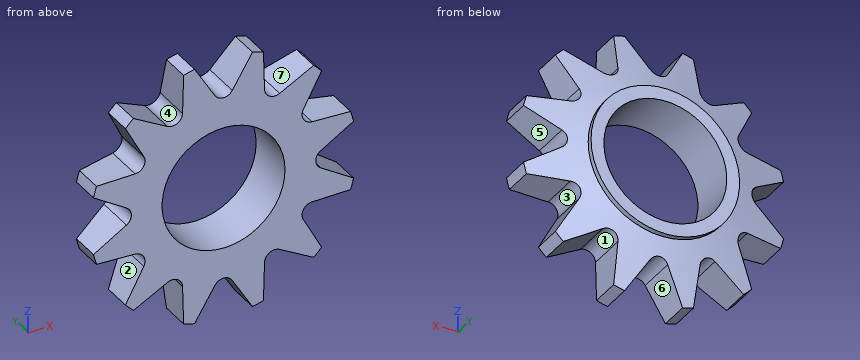
from build123d import *

# Parameters (mm, degrees)
SKETCH1_R               = 260
SKETCH1_R_2             = 120
BOSS_EXTRUDE1_DEPTH     = 45
SKETCH2_R               = 145
SKETCH2_R_2             = 120
BOSS_EXTRUDE3_DEPTH     = 55
CUT_EXTRUDE1_DEPTH      = 56
CUT_EXTRUDE1_DEPTH_BACK = 46
SCALE2_SCALE            = 0.4


with BuildPart() as part:
    # Sketch1 → Boss-Extrude1 (new body, symmetric)
    with BuildSketch(Plane(origin=(0, 0, 0), x_dir=(1, 0, 0), z_dir=(0, 1, 0))):
        Circle(SKETCH1_R)
        Circle(SKETCH1_R_2, mode=Mode.SUBTRACT)
    extrude(amount=BOSS_EXTRUDE1_DEPTH, both=True)

    # Sketch2 → Boss-Extrude3 (add)
    with BuildSketch(Plane(origin=(0, 0, 0), x_dir=(1, 0, 0), z_dir=(0, 1, 0))):
        Circle(SKETCH2_R)
        Circle(SKETCH2_R_2, mode=Mode.SUBTRACT)
    extrude(amount=BOSS_EXTRUDE3_DEPTH)

    # Sketch4 → Cut-Extrude1 (cut, two sides)
    with BuildSketch(Plane(origin=(0, 0, 0), x_dir=(1, 0, 0), z_dir=(0, 1, 0))) as cut_extrude1_sk:
        with BuildLine():
            Line((-17.033179487, 189.518072861), (-56.573051576, 253.770545642))
            ThreePointArc((-56.573051576, 253.770545642), (0, 260), (56.573051576, 253.770545642))
            Line((56.573051576, 253.770545642), (17.033179487, 189.518072861))
            ThreePointArc((17.033179487, 189.518072861), (0, 180), (-17.033179487, 189.518072861))
        make_face()
        with BuildLine():
            Line((109.510202574, 155.61087583), (175.878972656, 191.48521347))
            ThreePointArc((175.878972656, 191.48521347), (130, 225.166604984), (77.891572987, 248.058265046))
            Line((77.891572987, 248.058265046), (80.007870288, 172.644055317))
            ThreePointArc((80.007870288, 172.644055317), (90, 155.884572681), (109.510202574, 155.61087583))
        make_face()
        with BuildLine():
            Line((172.644055318, 80.007870287), (248.058265047, 77.891572986))
            ThreePointArc((248.058265047, 77.891572986), (225.166604985, 130), (191.485213471, 175.878972655))
            Line((191.485213471, 175.878972655), (155.610875831, 109.510202573))
            ThreePointArc((155.610875831, 109.510202573), (155.884572682, 90), (172.644055318, 80.007870287))
        make_face()
        with BuildLine():
            Line((189.518072862, -17.033179488), (253.770545643, -56.573051577))
            ThreePointArc((253.770545643, -56.573051577), (260.000000001, -1e-09), (253.770545643, 56.573051575))
            Line((253.770545643, 56.573051575), (189.518072862, 17.033179486))
            ThreePointArc((189.518072862, 17.033179486), (180.000000001, -1e-09), (189.518072862, -17.033179488))
        make_face()
        with BuildLine():
            Line((155.610875831, -109.510202575), (191.485213471, -175.878972657))
            ThreePointArc((191.485213471, -175.878972657), (225.166604985, -130.000000001), (248.058265047, -77.891572988))
            Line((248.058265047, -77.891572988), (172.644055318, -80.007870289))
            ThreePointArc((172.644055318, -80.007870289), (155.884572682, -90.000000001), (155.610875831, -109.510202575))
        make_face()
        with BuildLine():
            Line((80.007870288, -172.644055319), (77.891572987, -248.058265048))
            ThreePointArc((77.891572987, -248.058265048), (130, -225.166604986), (175.878972656, -191.485213472))
            Line((175.878972656, -191.485213472), (109.510202574, -155.610875832))
            ThreePointArc((109.510202574, -155.610875832), (90, -155.884572683), (80.007870288, -172.644055319))
        make_face()
        with BuildLine():
            Line((-17.033179487, -189.518072863), (-56.573051576, -253.770545644))
            ThreePointArc((-56.573051576, -253.770545644), (0, -260.000000002), (56.573051576, -253.770545644))
            Line((56.573051576, -253.770545644), (17.033179487, -189.518072863))
            ThreePointArc((17.033179487, -189.518072863), (0, -180.000000002), (-17.033179487, -189.518072863))
        make_face()
        with BuildLine():
            Line((-109.510202574, -155.610875832), (-175.878972656, -191.485213472))
            ThreePointArc((-175.878972656, -191.485213472), (-130, -225.166604986), (-77.891572987, -248.058265048))
            Line((-77.891572987, -248.058265048), (-80.007870288, -172.644055319))
            ThreePointArc((-80.007870288, -172.644055319), (-90, -155.884572683), (-109.510202574, -155.610875832))
        make_face()
        with BuildLine():
            Line((-172.644055318, -80.007870289), (-248.058265047, -77.891572988))
            ThreePointArc((-248.058265047, -77.891572988), (-225.166604985, -130.000000001), (-191.485213471, -175.878972657))
            Line((-191.485213471, -175.878972657), (-155.610875831, -109.510202575))
            ThreePointArc((-155.610875831, -109.510202575), (-155.884572682, -90.000000001), (-172.644055318, -80.007870289))
        make_face()
        with BuildLine():
            Line((-189.518072862, 17.033179486), (-253.770545643, 56.573051575))
            ThreePointArc((-253.770545643, 56.573051575), (-260.000000001, -1e-09), (-253.770545643, -56.573051577))
            Line((-253.770545643, -56.573051577), (-189.518072862, -17.033179488))
            ThreePointArc((-189.518072862, -17.033179488), (-180.000000001, -1e-09), (-189.518072862, 17.033179486))
        make_face()
        with BuildLine():
            Line((-155.610875831, 109.510202573), (-191.485213471, 175.878972655))
            ThreePointArc((-191.485213471, 175.878972655), (-225.166604985, 130), (-248.058265047, 77.891572986))
            Line((-248.058265047, 77.891572986), (-172.644055318, 80.007870287))
            ThreePointArc((-172.644055318, 80.007870287), (-155.884572682, 90), (-155.610875831, 109.510202573))
        make_face()
        with BuildLine():
            Line((-80.007870288, 172.644055317), (-77.891572987, 248.058265046))
            ThreePointArc((-77.891572987, 248.058265046), (-130, 225.166604984), (-175.878972656, 191.48521347))
            Line((-175.878972656, 191.48521347), (-109.510202574, 155.61087583))
            ThreePointArc((-109.510202574, 155.61087583), (-90, 155.884572681), (-80.007870288, 172.644055317))
        make_face()
    extrude(amount=CUT_EXTRUDE1_DEPTH, mode=Mode.SUBTRACT)
    extrude(cut_extrude1_sk.sketch, amount=-CUT_EXTRUDE1_DEPTH_BACK, mode=Mode.SUBTRACT)

    # Sketch9 → Cut-Revolve2 (revolve, cut)
    with BuildSketch(Plane(origin=(0, 0, 0), x_dir=(0, 0, -1), z_dir=(1, 0, 0))):
        Polygon((145, 45), (312.942286341, 45), (312.942286341, 0), align=None)
    revolve(axis=Axis((0, 0, 0), (0, 1, 0)), mode=Mode.SUBTRACT)


with BuildPart() as part_1:
    # Scale2: scaled about (-4.97e-06, -3.05192852, -9e-09)
    add(part.part.scale(SCALE2_SCALE).moved(Location((-2.982e-06, -1.831157112, -5e-09))))


solid = part_1.part
For this review, take the finished solid that the model builds, in its own axes (mm). Face numbers are marked on the shaded views. A direction names the side the tool comes from. Coordinates: 2 decimals unless noted, no trailing zeros. Loops run counter-clockwise (first coordinate to the right, second up) from the corner with the lowest first, then second, coordinate; pieces in that order, holes last. Notation, with made-up numbers: (63.25, -39.75) - (91.25, -39.75) arc R29 cw to (91.25, -19.75) - close; hole circle Ø8 at (-3, 16.25). An arc over 180 degrees is marked (long way). Use a Markdown table: item, result. Add a question column.
Item 1: Tool access review of the marked faces 5, 6 and 7: name each direction out of +Z, -Z, +X, -X, +Y, -Y from which nothing blocks a thin tool from reaching the whole face with its end or side.
Item 2: Insertion check: pin 1 Ø8 at (x, y) = (81, -6) entering from +Z; pin 2 Ø1 at (x, y) = (-10.5, 10) entering from -Z; pin 3 Ø3 at (x, y) = (50, -12) entering from -Z. Each pin has a flat end and moves straight along its axis. Give the tip position at first contact, or say it passes through.
Item 3: We need section A-A (z = 0). Give the boundary of the cut face in (x, y), and give its area (3 significant figures).
Item 4: Mouldability with a two-part tool opening along Z and no side actions: class the marked faces 1, 2, 3 and 4 as pulls with the +Z half, pulls with the -Z half, needs draft (parallel to the pull), parting line crosses it, or undercut.
Item 5: For line 1 (Z direction, x = -62, y = 3); line 2 (X direction, y = 4, z = 0); line 3 (X direction, y = 17, z = -24), list the stretches that pass through material, from the lowest coordinate up.
Results list:
| question | item | result |
|---|---|---|
| 1 | face 5 | +X, +Y, -Y |
| 1 | face 6 | -Z, +Y, -Y |
| 1 | face 7 | +Z, +Y, -Y |
| 2 | pin 1 | stops at z = 31.78 |
| 2 | pin 2 | stops at z = -82.08 |
| 2 | pin 3 | stops at z = -66.4 |
| 3 | outline | (-72, -19.83) - (-48, -19.83) - (-48, 20.17) - (-58, 20.17) - (-58, 16.17) - (-72, 12.42) - close; (48, -19.83) - (72, -19.83) - (72, 12.42) - (58, 16.17) - (58, 20.17) - (48, 20.17) - close |
| 3 | area | 1,760 mm^2 |
| 4 | face 1 | pulls with the -Z half |
| 4 | face 2 | undercut |
| 4 | face 3 | undercut |
| 4 | face 4 | pulls with the +Z half |
| 5 | line 1 | z = -72.08 to -43.31, -36.69 to 36.69, 43.31 to 72.08 |
| 5 | line 2 | x = -72 to -48, 48 to 72 |
| 5 | line 3 | x = -52.8 to -41.57, 41.57 to 52.8 |
